Source: CAD feature listing. Evaluate the final solid. Frame: model axes, mm. A direction names the side the tool comes from. Coordinates: 2 decimals unless noted, no trailing zeros. Order: outer loops, then holes, each group sorted by start corner. A loop starts at its lowest first (then second) coordinate and runs counter-clockwise, first axis right, second up.
Item 1: Contact query for flat-ended pins moving along their axis: P1, Ø0.8, axis at y = 16.5, z = 49, coming from the -X side; P2, Ø16, axis at x = 0, y = 51, coming from the -Z side; P3, Ø2.5, axis at y = 14.5, z = 1.5, coming from the +X side; P4, Ø1, axis at x = 6, z = 38.5, coming from the -Y side. Output: stop coordinate, or through.
Item 2: Reachability of faces 1 (the flat face through (-14, 14, 1)), 2 (the flat face through (1, -62.5, 25)), 3 (the flat face through (2, 1, 50)), 4 (the flat face through (14, 15, 1)) from +Z, -Z, +X, -X, +Y, -Y: full face, straight path, thin tool, end or side. Return the list, or none.
Item 3: Ray query, line 1 (Z direction, x = -4, y = 55.5); line 2 (Y direction, x = 0, z = 48.3); line 3 (Y direction, x = -1, z = 38). Return the intervals inside material, ascending.
Item 4: Mould query, pull axis Z, two halves, no side actions, for faces 5 (the cylindrical face through (10, 60.8, 48.8)), 6 (the flat face through (1, 0, 47.5)), 7 (the flat face through (0, 22, 0)). Classes: released by +Z, released by -Z, zero draft, split by the parting line, or undercut.
Item 5: Section B-B on x = -8. State how many separate pieces and enclosed holes the cut face has, then the cut area to 3 significant figures.
Item 6: Section A-A on y = 15. Return the cut outline in (x, z).
Item 7: Section C-C on y = -44. Return the cut outline in (x, z), then the cut area to 3 significant figures.
from build123d import *

# Parameters (mm, degrees)
ESBO_O1_W                  = 28
ESBO_O1_H                  = 130
RESSALTO_EXTRUS_O1_DEPTH   = 50
RESSALTO_EXTRUS_O2_START   = -50
ESBO_O2_R                  = 24
RESSALTO_EXTRUS_O2_DEPTH   = 50.000012
CORTE_EXTRUS_O2_DEPTH      = 86.782476988
CORTE_EXTRUS_O2_DEPTH_BACK = 86.782476988
ESBO_O6_W                  = 50
ESBO_O6_H                  = 3.715924279
CORTE_EXTRUS_O6_DEPTH      = 0.1
FILETE1_R                  = 14
CORTE_EXTRUS_O7_DEPTH      = 91.881514017
CORTE_EXTRUS_O8_DEPTH      = 91.881514017
ESBO_O12_R                 = 5
CORTE_EXTRUS_O10_DEPTH     = 86.782469994
ESBO_O13_R                 = 18
CORTE_EXTRUS_O11_DEPTH     = 86.782476988


with BuildPart() as part:
    # Esboço1 → Ressalto-extrusão1 (new body)
    with BuildSketch(Plane.XY):
        Rectangle(ESBO_O1_W, ESBO_O1_H)
    extrude(amount=RESSALTO_EXTRUS_O1_DEPTH)

    # Esboço2 → Ressalto-extrusão2 (add)
    with BuildSketch(Plane(origin=(0, 0, 0), x_dir=(-1, 0, 0), z_dir=(0, 0, -1)).offset(RESSALTO_EXTRUS_O2_START)):
        with Locations((-1.172051133, -41)):
            Circle(ESBO_O2_R)
    extrude(amount=RESSALTO_EXTRUS_O2_DEPTH)

    # Esboço5 → Corte-extrusão2 (cut, two sides: drawn at the far end of the back side and taken through both)
    with BuildSketch(Plane(origin=(0, 0, -1.2e-05), x_dir=(-1, 0, 0), z_dir=(0, 0, -1)).offset(-CORTE_EXTRUS_O2_DEPTH_BACK)):
        with BuildLine():
            ThreePointArc((-1.172051133, -65), (-7.844009292, -64.053957889), (-13.989971335, -61.290414528))
            Line((-13.989971335, -61.290414528), (-14, -65))
            Line((-14, -65), (-1.172051133, -65))
        make_face()
        with BuildLine():
            ThreePointArc((14, -59.595936771), (6.880821568, -63.608654123), (-1.172051133, -65))
            Line((-1.172051133, -65), (14, -65))
            Line((14, -65), (14, -59.595936771))
        make_face()
    extrude(amount=CORTE_EXTRUS_O2_DEPTH + CORTE_EXTRUS_O2_DEPTH_BACK, mode=Mode.SUBTRACT)

    # Esboço6 → Corte-extrusão6 (cut)
    with BuildSketch(Plane(origin=(14, 0, 0), x_dir=(0, 0, -1), z_dir=(1, 0, 0))):
        with Locations((-25, -63.14203786)):
            Rectangle(ESBO_O6_W, ESBO_O6_H)
    extrude(amount=-CORTE_EXTRUS_O6_DEPTH, mode=Mode.SUBTRACT)

    # Filete1
    filete1_edges = [part.edges().sort_by_distance(p)[0] for p in [
        (14, 65, 25),
        (-14, 65, 25),
    ]]
    fillet(filete1_edges, radius=FILETE1_R - 0.0001)  # a hair under: the kernel refuses the full size

    # Esboço8 → Corte-extrusão7 (cut, through all)
    with BuildSketch(Plane.ZY.offset(14)):
        Polygon((47.5, -22.404063229), (2.499991932, -22.404063229), (2.499988231, -62.5), (47.5, -62.5), align=None)
        Polygon((2.499998708, 51), (2.499991932, -22.404063229), (47.5, -22.404063229), (47.5, 51), align=None)
        Polygon((2.5, 64.999999769), (2.499998708, 51), (47.5, 51), (47.5, 65), align=None)
    extrude(amount=-CORTE_EXTRUS_O7_DEPTH, mode=Mode.SUBTRACT)

    # Esboço9 → Corte-extrusão8 (cut, through all)
    with BuildSketch(Plane(origin=(-14, 0, 0), x_dir=(0, 0, -1), z_dir=(1, 0, 0))):
        Polygon((-2.499991932, -22.404063229), (-2.499988499, -59.595936771), (-47.5, -59.595936771), (-47.5, -22.404063229), align=None)
    extrude(amount=-CORTE_EXTRUS_O8_DEPTH, mode=Mode.SUBTRACT)

    # Esboço12 → Corte-extrusão10 (cut, through all)
    with BuildSketch(Plane(origin=(0, 0, 0), x_dir=(-1, 0, 0), z_dir=(0, 0, -1))):
        with Locations((0, 51)):
            Circle(ESBO_O12_R)
    extrude(amount=-CORTE_EXTRUS_O10_DEPTH, mode=Mode.SUBTRACT)

    # Esboço13 → Corte-extrusão11 (cut, through all)
    with BuildSketch(Plane(origin=(0, 0, -1.2e-05), x_dir=(-1, 0, 0), z_dir=(0, 0, -1))):
        with Locations((-1.172051133, -41)):
            Circle(ESBO_O13_R)
    extrude(amount=-CORTE_EXTRUS_O11_DEPTH, mode=Mode.SUBTRACT)


solid = part.part
Answer list:
1. P1: stops at x = -14
1. P2: stops at z = 0
1. P3: stops at x = 14
1. P4: stops at y = -64.61
2. face 1: +Z, -Z, -X, +Y
2. face 2: +X, -X, +Y
2. face 3: +Z, +X, -X, +Y, -Y
2. face 4: +Z, -Z, +X, +Y
3. line 1: z = 0 to 2.5, 47.5 to 50
3. line 2: y = -64.97 to -58.96, -23.04 to 46, 56 to 65
3. line 3: y = -64.9 to -62.5
4. face 5: zero draft
4. face 6: undercut
4. face 7: released by -Z
5. separate pieces: 3
5. enclosed holes: 0
5. area: 504 mm2
6. outline: (-14, 0) - (14, 0) - (14, 2.5) - (-14, 2.5) - close; (-14, 47.5) - (14, 47.5) - (14, 50) - (-14, 50) - close
7. outline: (-22.64, 0) - (-16.58, 0) - (-16.58, 2.5) - (-22.64, 2.5) - close; (-22.64, 47.5) - (-16.58, 47.5) - (-16.58, 50) - (-22.64, 50) - close; (18.92, 0) - (24.98, 0) - (24.98, 2.5) - (18.92, 2.5) - close; (18.92, 47.5) - (24.98, 47.5) - (24.98, 50) - (18.92, 50) - close
7. area: 60.6 mm2
